CAD build for the part. Positions are in the model's coordinates, mm. Face numbers are marked on the shaded views. Round coordinates to 2 decimals unless told otherwise and drop trailing zeros. Loops run counter-clockwise (first coordinate to the right, second up) from the corner with the lowest first, then second, coordinate; pieces in that order, holes last.
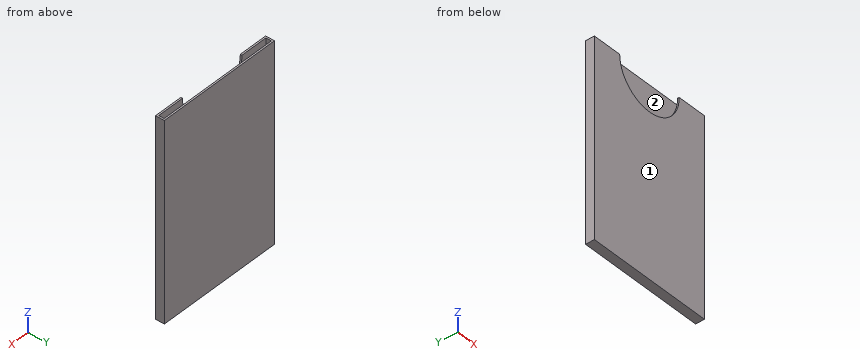
```python
from build123d import *

# Parameters (mm, degrees)
SKETCH_W        = 46.2
SKETCH_H        = 3.2
PAD_DEPTH       = 70.6
SKETCH001_W     = 45
SKETCH001_H     = 2
POCKET_DEPTH    = 70
SKETCH002_R     = 12.5
POCKET001_DEPTH = 0.6


with BuildPart() as part:
    # Sketch → Pad (new body)
    with BuildSketch(Plane.XY):
        with Locations((23.1, 1.6)):
            Rectangle(SKETCH_W, SKETCH_H)
    extrude(amount=PAD_DEPTH)

    # Sketch001 (on Face6 of Pad) → Pocket (cut)
    with BuildSketch(Plane.XY.offset(70.6)):
        with Locations((23.1, 1.6)):
            Rectangle(SKETCH001_W, SKETCH001_H)
    extrude(amount=-POCKET_DEPTH, mode=Mode.SUBTRACT)

    # Sketch002 (on Face6 of Pocket) → Pocket001 (cut)
    with BuildSketch(Plane.XZ):
        with Locations((23.1, 70.6)):
            Circle(SKETCH002_R)
    extrude(amount=-POCKET001_DEPTH, mode=Mode.SUBTRACT)


solid = part.part
```
Item 1: Flat gauge pins, fed straight in: P1, Ø1, axis at x = 37.5, y = 2, coming from the +Z side; P2, Ø4, axis at x = 28, z = 26.5, coming from the -Y side. Where does each tip first touch, or does it go through?
Answers follow:
P1: stops at z = 0.6
P2: stops at y = 0
Item 2: Cut at C-C, the plane x = 17. Give the cut face in (y, z), plus the area to 3 significant figures.
Answers follow:
outline: (0, 0) - (3.2, 0) - (3.2, 70.6) - (2.6, 70.6) - (2.6, 0.6) - (0.6, 0.6) - (0.6, 59.69) - (0, 59.69) - close
area: 79.4 mm2
Item 3: Probe line 1 (X direction, y = 2.2, z = 66); line 2 (Y direction, x = 15, z = 49.5); line 3 (Z direction, x = 9, y = 2.45). List the from-to ranges inside material, lowest first.
Answers follow:
line 1: x = 0 to 0.6, 45.6 to 46.2
line 2: y = 0 to 0.6, 2.6 to 3.2
line 3: z = 0 to 0.6
Item 4: Cut at B-B, the plane z = 48.5. Give the cut face in (x, y), plus the area to 3 significant figures.
Answers follow:
outline: (0, 0) - (46.2, 0) - (46.2, 3.2) - (0, 3.2) - close; hole (0.6, 0.6) - (45.6, 0.6) - (45.6, 2.6) - (0.6, 2.6) - close
area: 57.8 mm2
Item 5: Cut at A-A, the plane x = 27.5. Give the cut face in (y, z).
Answers follow:
outline: (0, 0) - (3.2, 0) - (3.2, 70.6) - (2.6, 70.6) - (2.6, 0.6) - (0.6, 0.6) - (0.6, 58.9) - (0, 58.9) - close
Item 6: Two-plate mould, pull along X, no slides. Class the marked faces 1 and 2: released by +X, released by -X, zero draft, split by the parting line, or undercut.
Answers follow:
face 1: zero draft
face 2: undercut
